Solid Edge part; units mm, degrees
sketch "Sketch1" plane through (0, 0, 0) normal (0, 0, 1) x (1, 0, 0)
  circle A0 centre (0, 0) radius 8.135
extrude "Protrusion1" add sketch "Sketch1" along normal blind 7
sketch "Sketch2" plane through (0, 0, 7) normal (0, 0, 1) x (1, 0, 0)
  line L0 (0, -2.8868) -> (-2.5, -1.4434)
  line L1 (-2.5, -1.4434) -> (-2.5, 1.4434)
  line L2 (-2.5, 1.4434) -> (0, 2.8868)
  line L3 (0, 2.8868) -> (2.5, 1.4434)
  line L4 (2.5, 1.4434) -> (2.5, -1.4434)
  line L5 (2.5, -1.4434) -> (0, -2.8868)
extrude "Cutout1" cut sketch "Sketch2" against normal blind 3.5
sketch "Sketch3" plane through (0, 0, 0) normal (0, 0, -1) x (0, 1, 0)
  circle A0 centre (0, 0) radius 5
extrude "Protrusion2" add sketch "Sketch3" along normal blind 25
sketch "Sketch4" plane through (0, 0, -25) normal (0, 0, -1) x (0, 1, 0)
  circle A0 centre (0, 0) radius 4
extrude "Protrusion3" add sketch "Sketch4" along normal blind 13
chamfer "Chamfer1" distance 0.5 angle 45 1 edges at (0, -4, -38)
properties part number "186231"
Build history of the part. All positions in model axes, mm. A direction names the side the tool comes from. Give positions to 0.01 mm unless a question says otherwise; leave off trailing zeros. Loops run counter-clockwise (first coordinate to the right, second up) from the corner with the lowest first, then second, coordinate; pieces in that order, holes last.
Item 1: Which spindle directions (+Z, -Z, +X, -X, +Y, -Y) get a long thin tool onto all of the face, cutting with end or side? Do faces 1 (the face through (3.905, -0.867, -31.162)), 2 (the face through (-1.764, 7.942, 3.451)), 3 (the face through (-1.267, 2.155, 5.274)). Say none if no direction does.
Answers follow:
face 1: -Z
face 2: +Z, -Z
face 3: +Z
Item 2: Slice it at B-B, the plane z = -17.5. List the corners of the cut face in (x, y).
Answers follow:
outline: circle Ø10 at (0, 0)
Item 3: Pull direction Y, two halves, no side cores. Call faces 4 (the face through (0, 0, -38)), 5 (the face through (4.88, -1.08, -12.32)), 6 (the face through (2.5, 0, 5)): released by +Y, released by -Y, zero draft, split by the parting line, or undercut.
Answers follow:
face 4: zero draft
face 5: split by the parting line
face 6: undercut
Item 4: Flat gauge pins, fed straight in: pin 1 (6 mm diameter, centred on x = 6, z = -22.5, fed in from -Y); pin 2 (1.5 mm diameter, centred on x = 1.5, z = -5, fed in from +Y); pin 3 (3 mm diameter, centred on x = -1.5, z = 0.5, fed in from -Y) (3 decimals); pin 4 (1 mm diameter, centred on x = -2.5, z = -17, fed in from -Y). Where does each tip first touch, or does it go through?
Answers follow:
pin 1: stops at y = -4
pin 2: stops at y = 4.94
pin 3: stops at y = -8.135
pin 4: stops at y = -4.58
Item 5: Drill centre lines: line 1 (Z direction, x = 7, y = 3.5); line 2 (Z direction, x = 0.5, y = -1.75); line 3 (X direction, y = 3, z = -5). Where is each one in solid material? Low to high.
Answers follow:
line 1: z = 0 to 7
line 2: z = -38 to 3.5
line 3: x = -4 to 4
Item 6: Slice it at C-C, the plane x = 4.5. List the corners of the cut face in (y, z).
Answers follow:
outline: (-6.78, 0) - (-2.18, 0) - (-2.18, -25) - (2.18, -25) - (2.18, 0) - (6.78, 0) - (6.78, 7) - (-6.78, 7) - close
Item 7: Slice it at D-D, the plane z = 3. List the corners of the cut face in (x, y) (3 decimals), and give its area (3 significant figures).
Answers follow:
outline: circle Ø16.27 at (0, 0)
area: 208 mm2
Item 8: Slice it at A-A, the plane y = 0. List the corners of the cut face in (x, z) (3 decimals).
Answers follow:
outline: (-8.135, 0) - (-5, 0) - (-5, -25) - (-4, -25) - (-4, -37.5) - (-3.5, -38) - (3.5, -38) - (4, -37.5) - (4, -25) - (5, -25) - (5, 0) - (8.135, 0) - (8.135, 7) - (2.5, 7) - (2.5, 3.5) - (-2.5, 3.5) - (-2.5, 7) - (-8.135, 7) - close
